from build123d import *

# Parameters (mm, degrees)
SKETCH1_R           = 2
BOSS_EXTRUDE1_DEPTH = 5
SKETCH2_W           = 14
SKETCH2_H           = 5
BOSS_EXTRUDE2_DEPTH = 14
SKETCH3_R           = 4
CUT_EXTRUDE1_DEPTH  = 25


with BuildPart() as part:
    # Sketch1 → Boss-Extrude1 (new body)
    with BuildSketch(Plane(origin=(0, 0, 0), x_dir=(0, 0, -1), z_dir=(1, 0, 0))):
        Polygon((61, 0), (75, 0), (75, 20), (-75, 20), (-75, 0), (-61, 0), (-61, 6), (61, 6), align=None)
        with Locations((-16, 13)):
            Circle(SKETCH1_R, mode=Mode.SUBTRACT)
        with Locations((-24, 13)):
            Circle(SKETCH1_R, mode=Mode.SUBTRACT)
        with Locations((-32, 13)):
            Circle(SKETCH1_R, mode=Mode.SUBTRACT)
        with Locations((-40, 13)):
            Circle(SKETCH1_R, mode=Mode.SUBTRACT)
        with Locations((16, 13)):
            Circle(SKETCH1_R, mode=Mode.SUBTRACT)
        with Locations((24, 13)):
            Circle(SKETCH1_R, mode=Mode.SUBTRACT)
        with Locations((32, 13)):
            Circle(SKETCH1_R, mode=Mode.SUBTRACT)
        with Locations((40, 13)):
            Circle(SKETCH1_R, mode=Mode.SUBTRACT)
        with Locations((-48, 13)):
            Circle(SKETCH1_R, mode=Mode.SUBTRACT)
        with Locations((-56, 13)):
            Circle(SKETCH1_R, mode=Mode.SUBTRACT)
        with Locations((-64, 13)):
            Circle(SKETCH1_R, mode=Mode.SUBTRACT)
        with Locations((48, 13)):
            Circle(SKETCH1_R, mode=Mode.SUBTRACT)
        with Locations((56, 13)):
            Circle(SKETCH1_R, mode=Mode.SUBTRACT)
        with Locations((64, 13)):
            Circle(SKETCH1_R, mode=Mode.SUBTRACT)
        with Locations((-8, 13)):
            Circle(SKETCH1_R, mode=Mode.SUBTRACT)
        with Locations((8, 13)):
            Circle(SKETCH1_R, mode=Mode.SUBTRACT)
    extrude(amount=BOSS_EXTRUDE1_DEPTH)

    # Sketch2 → Boss-Extrude2 (add)
    with BuildSketch(Plane.ZY):
        with Locations((-68, 2.5)):
            Rectangle(SKETCH2_W, SKETCH2_H)
        with Locations((68, 2.5)):
            Rectangle(SKETCH2_W, SKETCH2_H)
    extrude(amount=BOSS_EXTRUDE2_DEPTH)

    # Sketch3 → Cut-Extrude1 (cut)
    with BuildSketch(Plane(origin=(0, 0, 0), x_dir=(-1, 0, 0), z_dir=(0, -1, 0))):
        with Locations((7, -68)):
            Circle(SKETCH3_R)
        with Locations((7, 68)):
            Circle(SKETCH3_R)
    extrude(amount=-CUT_EXTRUDE1_DEPTH, mode=Mode.SUBTRACT)


solid = part.part
The listing builds one solid part. Answer for the finished solid, in the listing's coordinates (mm). A direction names the side the tool comes from. Coordinates: 2 decimals unless noted, no trailing zeros. Order: outer loops, then holes, each group sorted by start corner. A loop starts at its lowest first (then second) coordinate and runs counter-clockwise, first axis right, second up. Notation, with made-up numbers: (6.25, 2.25) -> (42.25, 2.25) arc R14 ccw to (42.25, 22.25) -> close; hole circle Ø9 at (-13.75, 36). An arc over 180 degrees is marked (long way). Answer in a Markdown table with one row per item. Add a question column.
Item 1: Each of these flat-tipped pins is pushed along its axis until it touches: P1, Ø4, axis at x = -7, z = -65.5, coming from the +Y side; P2, Ø4, axis at y = 12, z = -22.5, coming from the -X side; P3, Ø1.5, axis at x = 1.5, z = -28, coming from the -Y side. Where does it stop, or does it pass through?
Item 2: Find section B-B (x = -7). Write down the section's boundary in (y, z), then the cut area to 3 significant figures.
Item 3: Determine the mould class of faces 3 (the face through (-14, 3, 68)), 4 (the face through (2.465, 14.352, -46.526)), 5 (the face through (-10, 5, -71)) for opening direction Y: +Y half, -Y half, draft (parallel to the pull), parting line (faces both ways), or undercut.
Item 4: Find the intervals of material crossed by L1, parallel to X at y = 2, z = -68; L2, parallel to Y at x = 3.5, z = 64; L3, parallel to X at y = 17, z = 16.5, in increasing order. Write a range as from..to.
Item 5: Find section A-A (z = 68). Write down the section's boundary in (x, y).
Item 6: Find section C-C (y = 1.25). Write down the section's boundary in (x, z), then the cut area to 3 significant figures.
Item 7: Find section D-D (z = -48). Write down the section's boundary in (x, y), then the cut area to 3 significant figures.
Item 8: Which of the six approach directions +Z, -Z, +X, -X, +Y, -Y give full straight-line access (tool end or side, diameter ignored) to faces 1 (the face through (2.465, 14.352, -38.526)), 2 (the face through (-5, 3, 61))?
Result set:
| question | item | result |
|---|---|---|
| 1 | P1 | stops at y = 5 |
| 1 | P2 | stops at x = 0 |
| 1 | P3 | stops at y = 6 |
| 2 | outline | (0, -75) -> (5, -75) -> (5, -72) -> (0, -72) -> close; (0, -64) -> (5, -64) -> (5, -61) -> (0, -61) -> close; (0, 61) -> (5, 61) -> (5, 64) -> (0, 64) -> close; (0, 72) -> (5, 72) -> (5, 75) -> (0, 75) -> close |
| 2 | area | 60.0 mm² |
| 3 | face 3 | draft |
| 3 | face 4 | undercut |
| 3 | face 5 | +Y half |
| 4 | L1 | x = -14..-11, -3..5 |
| 4 | L2 | y = 0..11, 15..20 |
| 4 | L3 | x = 0..5 |
| 5 | outline | (-14, 0) -> (-11, 0) -> (-11, 5) -> (-14, 5) -> close; (-3, 0) -> (5, 0) -> (5, 20) -> (0, 20) -> (0, 5) -> (-3, 5) -> close |
| 6 | outline | (-14, -75) -> (5, -75) -> (5, -61) -> (-14, -61) -> close; (-14, 61) -> (5, 61) -> (5, 75) -> (-14, 75) -> close; hole circle Ø8 at (-7, -68); hole circle Ø8 at (-7, 68) |
| 6 | area | 431 mm² |
| 7 | outline | (0, 6) -> (5, 6) -> (5, 11) -> (0, 11) -> close; (0, 15) -> (5, 15) -> (5, 20) -> (0, 20) -> close |
| 7 | area | 50.0 mm² |
| 8 | face 1 | +X, -X |
| 8 | face 2 | +X, -X, -Y |
